```python
from build123d import *

# Parameters (mm, degrees)
SKETCH1_R                                         = 2.5
BOSS_EXTRUDE1_DEPTH                               = 5
BOSS_EXTRUDE1_2_DEPTH                             = 5
BOSS_EXTRUDE1_3_DEPTH                             = 5
BOSS_EXTRUDE1_4_DEPTH                             = 5
SKETCH3_W                                         = 77.6
SKETCH3_H                                         = 61.3
BOSS_EXTRUDE2_DEPTH                               = 3
SKETCH4_W                                         = 77.6
SKETCH4_H                                         = 61.3
SKETCH4_W_2                                       = 73.6
SKETCH4_H_2                                       = 57.3
BOSS_EXTRUDE3_DEPTH                               = 25
CUT_EXTRUDE2_REACH                                = 87.797
SKETCH5_W                                         = 13.5
SKETCH5_H                                         = 13
SKETCH5_W_2                                       = 11.5
FILLET1_R                                         = 1
SKETCH7_W                                         = 75.2
SKETCH7_H                                         = 58.9
CUT_EXTRUDE3_DEPTH                                = 2
SKETCH2_R                                         = 1
CUT_EXTRUDE1_DEPTH                                = 55.069053071
CSK_FOR_M2_5_FLAT_HEAD_MACHINE_SCREW1_D           = 2.9
CSK_FOR_M2_5_FLAT_HEAD_MACHINE_SCREW1_CSINK_D     = 5.5
CSK_FOR_M2_5_FLAT_HEAD_MACHINE_SCREW1_CSINK_ANGLE = 90
SKETCH12_R                                        = 3.1
CUT_EXTRUDE4_DEPTH                                = 2
FILLET3_R                                         = 1
FILLET4_R                                         = 1


with BuildPart() as part:
    # Sketch1 → Boss-Extrude1 (new body)
    with BuildSketch(Plane(origin=(0, 0, 0), x_dir=(1, 0, 0), z_dir=(0, 1, 0))):
        with Locations(Location((-32.6, 19.09, 0), (0, 0, 270))):
            Circle(SKETCH1_R)
    extrude(amount=-BOSS_EXTRUDE1_DEPTH)



with BuildPart() as body_2:
    # Sketch1 → Boss-Extrude1 2 (new body)
    with BuildSketch(Plane(origin=(0, 0, 0), x_dir=(1, 0, 0), z_dir=(0, 1, 0))):
        with Locations(Location((-32.6, -8.85, 0), (0, 0, 270))):
            Circle(SKETCH1_R)
    extrude(amount=-BOSS_EXTRUDE1_2_DEPTH)


with BuildPart() as body_3:
    # Sketch1 → Boss-Extrude1 3 (new body)
    with BuildSketch(Plane(origin=(0, 0, 0), x_dir=(1, 0, 0), z_dir=(0, 1, 0))):
        with Locations(Location((19.8, 24.15, 0), (0, 0, 270))):
            Circle(SKETCH1_R)
    extrude(amount=-BOSS_EXTRUDE1_3_DEPTH)


with BuildPart() as body_4:
    # Sketch1 → Boss-Extrude1 4 (new body)
    with BuildSketch(Plane(origin=(0, 0, 0), x_dir=(1, 0, 0), z_dir=(0, 1, 0))):
        with Locations(Location((18.5, -24.05, 0), (0, 0, 270))):
            Circle(SKETCH1_R)
    extrude(amount=-BOSS_EXTRUDE1_4_DEPTH)


with BuildPart() as part_1:
    add(part.part)

    add(body_2.part)  # Boss-Extrude2 merges body 2

    add(body_3.part)  # Boss-Extrude2 merges body 3

    add(body_4.part)  # Boss-Extrude2 merges body 4
    # Sketch3 → Boss-Extrude2 (add)
    with BuildSketch(Plane.XZ.offset(5)):
        with Locations((-1, 0)):
            Rectangle(SKETCH3_W, SKETCH3_H)
    extrude(amount=BOSS_EXTRUDE2_DEPTH)

    # Sketch4 → Boss-Extrude3 (add)
    with BuildSketch(Plane(origin=(0, -5, 0), x_dir=(1, 0, 0), z_dir=(0, 1, 0))):
        with Locations((-1, 0)):
            Rectangle(SKETCH4_W, SKETCH4_H)
        with Locations((-1, 0)):
            Rectangle(SKETCH4_W_2, SKETCH4_H_2, mode=Mode.SUBTRACT)
    extrude(amount=BOSS_EXTRUDE3_DEPTH)

    # Sketch5 → Cut-Extrude2 (cut, up to next)
    with BuildSketch(Plane(origin=(37.8, 0, 0), x_dir=(0, 0, -1), z_dir=(1, 0, 0)), mode=Mode.PRIVATE) as cut_extrude2_sk1:
        with Locations((-11.45, 7.5)):
            Rectangle(SKETCH5_W, SKETCH5_H)
    cut_extrude2_tool1 = extrude(cut_extrude2_sk1.sketch, amount=-CUT_EXTRUDE2_REACH, mode=Mode.PRIVATE) & part_1.part
    # Sketch5 → Cut-Extrude2 (cut, up to next)
    with BuildSketch(Plane(origin=(37.8, 0, 0), x_dir=(0, 0, -1), z_dir=(1, 0, 0)), mode=Mode.PRIVATE) as cut_extrude2_sk2:
        with Locations((17.9, 7.5)):
            Rectangle(SKETCH5_W_2, SKETCH5_H)
    cut_extrude2_tool2 = extrude(cut_extrude2_sk2.sketch, amount=-CUT_EXTRUDE2_REACH, mode=Mode.PRIVATE) & part_1.part
    add(cut_extrude2_tool1.solids().sort_by_distance((37.8, 7.5, 11.45))[0], mode=Mode.SUBTRACT)
    add(cut_extrude2_tool2.solids().sort_by_distance((37.8, 7.5, -17.9))[0], mode=Mode.SUBTRACT)

    # Fillet1
    fillet1_edges = [part_1.edges().sort_by_distance(p)[0] for p in [
        (-1, -5, 28.65),
        (-1, -5, -28.65),
        (-37.8, -5, 0),
        (35.8, 7.5, -28.65),
        (-37.8, 7.5, -28.65),
        (-37.8, 7.5, 28.65),
        (35.8, 7.5, 28.65),
        (37.8, -8, 0),
    ]]
    fillet(fillet1_edges, radius=FILLET1_R)

    # Sketch7 → Cut-Extrude3 (cut)
    with BuildSketch(Plane(origin=(0, 20, 0), x_dir=(1, 0, 0), z_dir=(0, 1, 0))):
        with Locations((-1, 0)):
            Rectangle(SKETCH7_W, SKETCH7_H)
    extrude(amount=-CUT_EXTRUDE3_DEPTH, mode=Mode.SUBTRACT)

    # Sketch2 → Cut-Extrude1 (cut, through all)
    with BuildSketch(Plane(origin=(0, 0, 0), x_dir=(1, 0, 0), z_dir=(0, 1, 0))):
        with Locations(Location((-32.6, -8.85, 0), (0, 0, 270))):
            Circle(SKETCH2_R)
        with Locations(Location((-32.6, 19.09, 0), (0, 0, 270))):
            Circle(SKETCH2_R)
        with Locations(Location((19.8, 24.15, 0), (0, 0, 270))):
            Circle(SKETCH2_R)
        with Locations(Location((18.5, -24.05, 0), (0, 0, 270))):
            Circle(SKETCH2_R)
    extrude(amount=-CUT_EXTRUDE1_DEPTH, mode=Mode.SUBTRACT)

    # CSK for M2.5 Flat Head Machine Screw1 (through all)
    with Locations(Plane(origin=(0, -8, 0), x_dir=(-1, 0, 0), z_dir=(0, -1, 0))):
        with Locations((32.6, 19.09), (32.6, -8.85), (-18.5, -24.05), (-19.8, 24.15)):
            CounterSinkHole(CSK_FOR_M2_5_FLAT_HEAD_MACHINE_SCREW1_D / 2, CSK_FOR_M2_5_FLAT_HEAD_MACHINE_SCREW1_CSINK_D / 2, counter_sink_angle=CSK_FOR_M2_5_FLAT_HEAD_MACHINE_SCREW1_CSINK_ANGLE)

    # Sketch12 → Cut-Extrude4 (cut)
    with BuildSketch(Plane.ZY.offset(39.8)):
        with Locations((16.65, 10)):
            Circle(SKETCH12_R)
    extrude(amount=-CUT_EXTRUDE4_DEPTH, mode=Mode.SUBTRACT)

    # Fillet3
    fillet3_edges = [part_1.edges().sort_by_distance(p)[0] for p in [
        (-39.8, 6, 30.65),
        (-39.8, 6, -30.65),
        (-1.5, -8, -30.65),
        (-1.5, -8, 30.65),
        (37.8, 6.5, 30.65),
        (37.507106781, -7.707106781, 30.65),
        (37.8, 6.5, -30.65),
        (37.507106781, -7.707106781, -30.65),
    ]]
    fillet(fillet3_edges, radius=FILLET3_R)

    # Fillet4
    # the kernel refuses this fillet: 1 mm, written as the material it takes off along each edge
    with BuildSketch(Plane(origin=(-38.8, -7, -29.65), x_dir=(0, -1, 0), z_dir=(-1, 0, 0))) as fillet4_piece_1_section:
        Polygon((0, 0), (FILLET4_R, 0), (FILLET4_R, -FILLET4_R), (0, -FILLET4_R), align=None)
    fillet4_piece_1 = extrude(amount=FILLET4_R, mode=Mode.PRIVATE)
    fillet4_piece_1 = fillet4_piece_1 - Plane(origin=(-38.8, -7, -29.65), x_dir=(0, 0.7071067811865475, 0.7071067811865475), z_dir=(-1, 0, 0)) * Sphere(FILLET4_R, mode=Mode.PRIVATE)
    add(fillet4_piece_1, mode=Mode.SUBTRACT)
    with BuildSketch(Plane(origin=(-38.8, -7, 29.65), x_dir=(0, -1, 0), z_dir=(-1, 0, 0))) as fillet4_piece_2_section:
        Polygon((0, 0), (FILLET4_R, 0), (FILLET4_R, FILLET4_R), (0, FILLET4_R), align=None)
    fillet4_piece_2 = extrude(amount=FILLET4_R, mode=Mode.PRIVATE)
    fillet4_piece_2 = fillet4_piece_2 - Plane(origin=(-38.8, -7, 29.65), x_dir=(0, 0.7071067811865475, -0.7071067811865475), z_dir=(-1, 0, 0)) * Sphere(FILLET4_R, mode=Mode.PRIVATE)
    add(fillet4_piece_2, mode=Mode.SUBTRACT)
    with BuildSketch(Plane(origin=(-39.8, -8, -29.65), x_dir=(0, 1, 0), z_dir=(0, 0, 1))) as fillet4_piece_3:
        with BuildLine():
            CenterArc((FILLET4_R, -FILLET4_R), FILLET4_R, 90, 90)
            Line((0, -FILLET4_R), (0, 0))
            Line((0, 0), (FILLET4_R, 0))
        make_face()
    extrude(amount=59.3, mode=Mode.SUBTRACT)


solid = part_1.part
```
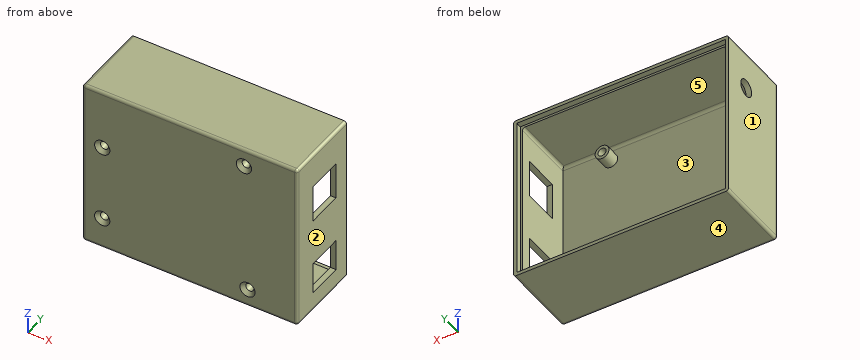
The listing builds one solid part. Answer for the finished solid, in the listing's coordinates (mm). Face numbers are marked on the shaded views. A direction names the side the tool comes from. Give positions to 0.01 mm unless a question says otherwise; leave off trailing zeros. Order: outer loops, then holes, each group sorted by start corner. A loop starts at its lowest first (then second) coordinate and runs counter-clockwise, first axis right, second up.
1) Find section C-C on y = -2.5. Give the number of separate pieces and of enclosed holes in the cut face, then the cut area to 3 significant figures.
Reported:
separate pieces: 5
enclosed holes: 5
area: 592 mm2
2) Determine the mould class of the marked faces 1, 2 and 3 for opening direction X: pulls with the +X half, pulls with the -X half, needs draft (parallel to the pull), parting line crosses it, or undercut.
Reported:
face 1: pulls with the -X half
face 2: pulls with the +X half
face 3: undercut
3) For the marked faces 4 and 5, determine the directions among +Z, -Z, +X, -X, +Y, -Y from which every point of the face is accessible in a straight line to the end or side of a thin tool.
Reported:
face 4: -Z, +X, -X, +Y, -Y
face 5: +Y
4) Find section A-A on y = 5.25. Write down the section's boundary in (x, z).
Reported:
outline: (-39.8, -29.65) arc R1 ccw to (-38.8, -30.65) - (36.8, -30.65) arc R1 ccw to (37.8, -29.65) - (37.8, -23.65) - (35.8, -23.65) - (35.8, -27.65) arc R1 cw to (34.8, -28.65) - (-36.8, -28.65) arc R1 cw to (-37.8, -27.65) - (-37.8, 27.65) arc R1 cw to (-36.8, 28.65) - (34.8, 28.65) arc R1 cw to (35.8, 27.65) - (35.8, 18.2) - (37.8, 18.2) - (37.8, 29.65) arc R1 ccw to (36.8, 30.65) - (-38.8, 30.65) arc R1 ccw to (-39.8, 29.65) - close; (35.8, -12.15) - (37.8, -12.15) - (37.8, 4.7) - (35.8, 4.7) - close
5) Given P1, Ø16.5, axis at x = -9.5, z = -10, coming from the +Y side; P2, Ø8, axis at y = 10, z = 16.65, coming from the -X side; P3, Ø4, axis at x = 18.5, z = 24.05, coming from the -Y side; P4, Ø3.5, axis at x = 19.8, z = -24.15, coming from the -Y side, each flat-ended and moving along its own axis, determine where each tip first touches the part or whether it passes through.
Reported:
P1: stops at y = -5
P2: stops at x = -39.8
P3: stops at y = -7.25
P4: stops at y = -7
6) Find section B-B on z = 24.05. Write down the section's boundary in (x, y).
Reported:
outline: (-39.8, -7) arc R1 ccw to (-38.8, -8) - (15.75, -8) - (17.05, -6.7) - (17.05, 0) - (16, 0) - (16, -5) - (-36.8, -5) arc R1 cw to (-37.8, -4) - (-37.8, 18) - (-38.6, 18) - (-38.6, 20) - (-39.8, 20) - close; (19.95, -6.7) - (21.25, -8) - (36.8, -8) arc R1 ccw to (37.8, -7) - (37.8, 20) - (36.6, 20) - (36.6, 18) - (35.8, 18) - (35.8, -5) - (21, -5) - (21, 0) - (19.95, 0) - close
7) Consider line 1 along X through (y, z) = (12.75, 2); line 2 along X through (y, z) = (-2.75, 24.5); line 3 along Z through (x, y) = (-4.5, -0.75). Determine where each line is inside the solid, lowest interval first.
Reported:
line 1: x = -39.8 to -37.8, 35.8 to 37.8
line 2: x = -39.8 to -37.8, 16.04 to 17.12, 19.88 to 20.96, 35.8 to 37.8
line 3: z = -30.65 to -28.65, 28.65 to 30.65
